from build123d import *

# Parameters (mm, degrees)
BOSS_EXTRUDE1_DEPTH     = 12.7
SKETCH10_R              = 3.082136138
CUT_EXTRUDE1_DEPTH      = 26.185474767
SKETCH11_W              = 2.435876878
SKETCH11_H              = 7.908405343
CUT_EXTRUDE2_DEPTH      = 26.185474767
CUT_EXTRUDE4_DEPTH      = 31.460304214
CUT_EXTRUDE4_DEPTH_BACK = 31.460304214
SKETCH13_W              = 5.182015338
SKETCH13_H              = 2.489456313
FILLET3_R               = 0.508
SKETCH17_W              = 0.605016918
SKETCH17_H              = 2.095446093
SKETCH17_W_2            = 0.604461085
SKETCH17_H_2            = 2.141007526
CUT_EXTRUDE7_DEPTH      = 26.185474767
SKETCH19_W              = 12.7
SKETCH19_H              = 6.295576116
BOSS_EXTRUDE2_DEPTH     = 3.048
SKETCH20_W              = 12.7
SKETCH20_H              = 6.295576116
BOSS_EXTRUDE3_DEPTH     = 2.0066
SKETCH22_W              = 5.182015338
SKETCH22_H              = 2.489456313
CUT_EXTRUDE8_DEPTH      = 35.014712144


with BuildPart() as part:
    # Sketch5 → Boss-Extrude1 (new body)
    with BuildSketch(Plane.XY):
        Polygon((-6.474794456, -10.4902), (-6.938297275, -10.378313453), (-7.308763147, -10.05450356), (-7.490794456, -9.4742), (-7.378907909, -9.01069718), (-7.193214945, -8.75577951), (-3.863171405, -5.42573597), (-2.833127272, -4.737482484), (-1.618107374, -4.4958), (1.618107374, -4.4958), (2.668236067, -4.674493152), (3.863171405, -5.42573597), (7.193214945, -8.75577951), (7.490794456, -9.4742), (7.378907909, -9.93770282), (6.938297275, -10.378313453), (6.474794456, -10.4902), (4.3434, -10.4902), (3.646537163, -10.737670005), (3.377082754, -11.059343535), (3.2385, -11.5951), (3.485970005, -12.291962837), (3.807643535, -12.561417246), (4.3434, -12.7), (10.5918, -12.7), (10.5918, -18.995576116), (-9.5504, -18.995576116), (-9.5504, -12.7), (-4.3434, -12.7), (-3.863171405, -12.590180165), (-3.485969976, -12.291962837), (-3.271081829, -11.861441531), (-3.271081829, -11.328758469), (-3.485969976, -10.898237163), (-3.863171405, -10.600019835), (-4.3434, -10.4902), align=None)
    extrude(amount=-BOSS_EXTRUDE1_DEPTH)

    # Sketch10 → Cut-Extrude1 (cut, through all)
    with BuildSketch(Plane.XY):
        with Locations((-0.066530556, -6.095976424)):
            Circle(SKETCH10_R)
    extrude(amount=-CUT_EXTRUDE1_DEPTH, mode=Mode.SUBTRACT)

    # Sketch11 → Cut-Extrude2 (cut, through all)
    with BuildSketch(Plane.XY):
        with Locations((0, -9.781904855)):
            Rectangle(SKETCH11_W, SKETCH11_H)
    extrude(amount=-CUT_EXTRUDE2_DEPTH, mode=Mode.SUBTRACT)

    # Sketch13 → Cut-Extrude4 (cut, two sides: drawn at the far end of the back side and taken through both)
    with BuildSketch(Plane.ZY.offset(9.5504).offset(-CUT_EXTRUDE4_DEPTH_BACK)):
        with Locations((-6.35, -15.847788058)):
            Rectangle(SKETCH13_W, SKETCH13_H)
    extrude(amount=CUT_EXTRUDE4_DEPTH + CUT_EXTRUDE4_DEPTH_BACK, mode=Mode.SUBTRACT)

    # Fillet3
    # the kernel refuses this fillet: 0.508 mm, written as the material it takes off along each edge
    with BuildSketch(Plane(origin=(2.668236067, -4.674493152, 3.28944818), x_dir=(0.8465916632907231, -0.5322429479538896, 0), z_dir=(0, 0, -1))) as fillet3_piece_1:
        with BuildLine():
            CenterArc((1.315779272, 0.508), FILLET3_R, 143.192029884, 126.807970116)
            Line((0.90905007, 0.812360569), (0.900915486, 0.81844778))
            ThreePointArc((0.900915486, 0.81844778), (0.488321858, 0.368360866), (-0.005137978, 0.008765089))
            Line((-0.005137978, 0.008765089), (0, -0.01016))
            Line((0, -0.01016), (1.315779272, -0.01016))
            Line((1.315779272, -0.01016), (1.315779272, 0))
        make_face()
    extrude(amount=19.278896361, mode=Mode.SUBTRACT)
    with BuildSketch(Plane(origin=(-2.833127272, -4.737482484, 3.097058862), x_dir=(-0.2544986167721869, -0.9670731379068719, 0), z_dir=(0, 0, -1))) as fillet3_piece_2:
        with BuildLine():
            CenterArc((1.319821852, 0.497962426), FILLET3_R, 140.517787887, 118.073467257)
            Line((0.927736265, 0.820968451), (0.919894553, 0.827428572))
            ThreePointArc((0.919894553, 0.827428572), (0.4571351, 0.418092896), (-0.006733033, 0.007608671))
            Line((-0.006733033, 0.007608671), (0.002009719, -0.009959249))
            ThreePointArc((0.002009719, -0.009959249), (0.60966796, 0.050739942), (1.217326201, -0.009959249))
            Line((1.217326201, -0.009959249), (1.219335919, 0))
        make_face()
    extrude(amount=18.894117724, mode=Mode.SUBTRACT)

    # Sketch17 → Cut-Extrude7 (cut, through all)
    with BuildSketch(Plane.XY):
        with Locations((3.55718824, -12.68838448)):
            Rectangle(SKETCH17_W, SKETCH17_H)
        with Locations((-3.573312372, -12.665603763)):
            Rectangle(SKETCH17_W_2, SKETCH17_H_2)
    extrude(amount=-CUT_EXTRUDE7_DEPTH, mode=Mode.SUBTRACT)

    # Sketch19 → Boss-Extrude2 (add)
    with BuildSketch(Plane.ZY.offset(9.5504)):
        with Locations((-6.35, -15.847788058)):
            Rectangle(SKETCH19_W, SKETCH19_H)
    extrude(amount=BOSS_EXTRUDE2_DEPTH)

    # Sketch20 → Boss-Extrude3 (add)
    with BuildSketch(Plane(origin=(10.5918, 0, 0), x_dir=(0, 0, -1), z_dir=(1, 0, 0))):
        with Locations((6.35, -15.847788058)):
            Rectangle(SKETCH20_W, SKETCH20_H)
    extrude(amount=BOSS_EXTRUDE3_DEPTH)

    # Sketch22 → Cut-Extrude8 (cut, through all)
    with BuildSketch(Plane.ZY.offset(12.5984)):
        with Locations((-6.35, -15.847788058)):
            Rectangle(SKETCH22_W, SKETCH22_H)
    extrude(amount=-CUT_EXTRUDE8_DEPTH, mode=Mode.SUBTRACT)


solid = part.part
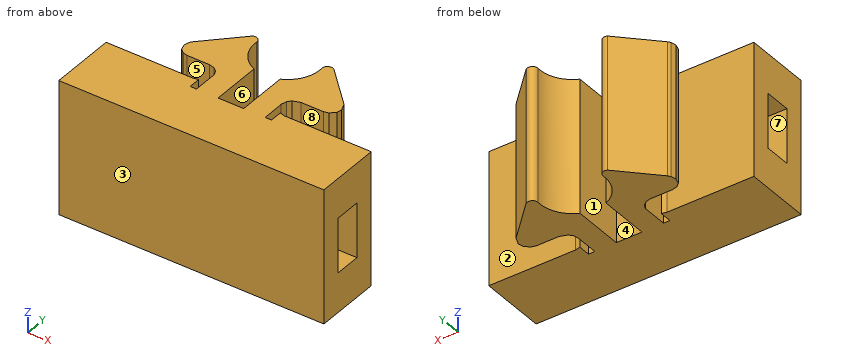
Work out the finished part from the listing and answer in its coordinate system (mm). Face numbers are marked on the shaded views. A direction names the side the tool comes from. Give positions to 0.01 mm unless a question says otherwise; leave off trailing zeros. Loops run counter-clockwise (first coordinate to the right, second up) from the corner with the lowest first, then second, coordinate; pieces in that order, holes last. Notation, with made-up numbers: (-34.5, 50) - (20.5, 50) arc R16 cw to (20.5, 69) - close; hole circle Ø9 at (-37, -1). An arc over 180 degrees is marked (long way). Answer in a Markdown table with one row per item. Add a question column.
Q1. Consider line 1 along X through (y, z) = (-12.5, -8.75); line 2 along Z through (x, y) = (7.25, -15.25); line 3 along Y through (x, z) = (-5, -4.25). Determine where each line is inside the solid, lowest interval first.
Q2. Determine the mould class of the marked faces 1, 2, 3 and 4 for opening direction Y: released by +Y, released by -Y, zero draft, split by the parting line, or undercut.
Q3. The part is cut by section C-C (x = 0). Determine the outline of the cut face in (y, z).
Q4. Each of these flat-tipped pins is pushed along its axis until it touches: P1, Ø6.5, axis at x = 8, z = -4.5, coming from the +Y side; P2, Ø5, axis at y = -8, z = -8, coming from the -X side; P3, Ø1.5, axis at x = -5, z = -2, coming from the +Y side. Where does it stop, or does it pass through?
Q5. A tool of negligible diameter and unlimited length cuts with its end or side. For the marked faces 5, 6, 7 and 8, from which of +Z, -Z, +X, -X, +Y, -Y can it reach the whole face along a straight path? Write none if from no direction.
Q6. The part is cut by section D-D (x = -8.75). Determine the outline of the cut face in (y, z), and give its area (3 significant figures).
Q7. The part is cut by section B-B (y = -13). Determine the outline of the cut face in (x, z), and give its area (3 significant figures).
Q8. The part is cut by section A-A (y = -15.25). Determine the outline of the cut face in (x, z).
Solution:
| question | item | result |
|---|---|---|
| 1 | line 1 | x = -3.27 to -1.22, 1.22 to 3.25 |
| 1 | line 2 | z = -12.7 to -8.94, -3.76 to 0 |
| 1 | line 3 | y = -19 to -17.09, -14.6 to -12.7, -10.49 to -6.56 |
| 2 | face 1 | zero draft |
| 2 | face 2 | undercut |
| 2 | face 3 | released by -Y |
| 2 | face 4 | released by +Y |
| 3 | outline | (-19, -12.7) - (-13.74, -12.7) - (-13.74, 0) - (-19, 0) - close; hole (-17.09, -8.94) - (-14.6, -8.94) - (-14.6, -3.76) - (-17.09, -3.76) - close |
| 4 | P1 | stops at y = -6.31 |
| 4 | P2 | stops at x = -7.49 |
| 4 | P3 | stops at y = -5.81 |
| 5 | face 5 | +Z, -Z, -X |
| 5 | face 6 | +Z, -Z, +Y |
| 5 | face 7 | +X, -X |
| 5 | face 8 | +Z, -Z, +X |
| 6 | outline | (-19, -12.7) - (-12.7, -12.7) - (-12.7, 0) - (-19, 0) - close; hole (-17.09, -8.94) - (-14.6, -8.94) - (-14.6, -3.76) - (-17.09, -3.76) - close |
| 6 | area | 67.1 mm² |
| 7 | outline | (-12.6, -12.7) - (-3.88, -12.7) - (-3.88, 0) - (-12.6, 0) - close; (-3.27, -12.7) - (-1.22, -12.7) - (-1.22, 0) - (-3.27, 0) - close; (1.22, -12.7) - (3.25, -12.7) - (3.25, 0) - (1.22, 0) - close; (3.86, -12.7) - (12.6, -12.7) - (12.6, 0) - (3.86, 0) - close |
| 7 | area | 274 mm² |
| 8 | outline | (-12.6, -12.7) - (12.6, -12.7) - (12.6, -8.94) - (-12.6, -8.94) - close; (-12.6, -3.76) - (12.6, -3.76) - (12.6, 0) - (-12.6, 0) - close |
